Study the drawing (mm; zero at the part's minimum x, y, z) and answer. A direction names the side the tool comes from. Coordinates: 2 decimals unless noted, no trailing zeros. Order: outer loops, then holes, each group sorted by start corner. A loop starts at its lowest first (then second) coordinate and runs counter-clockwise, first axis right, second up.
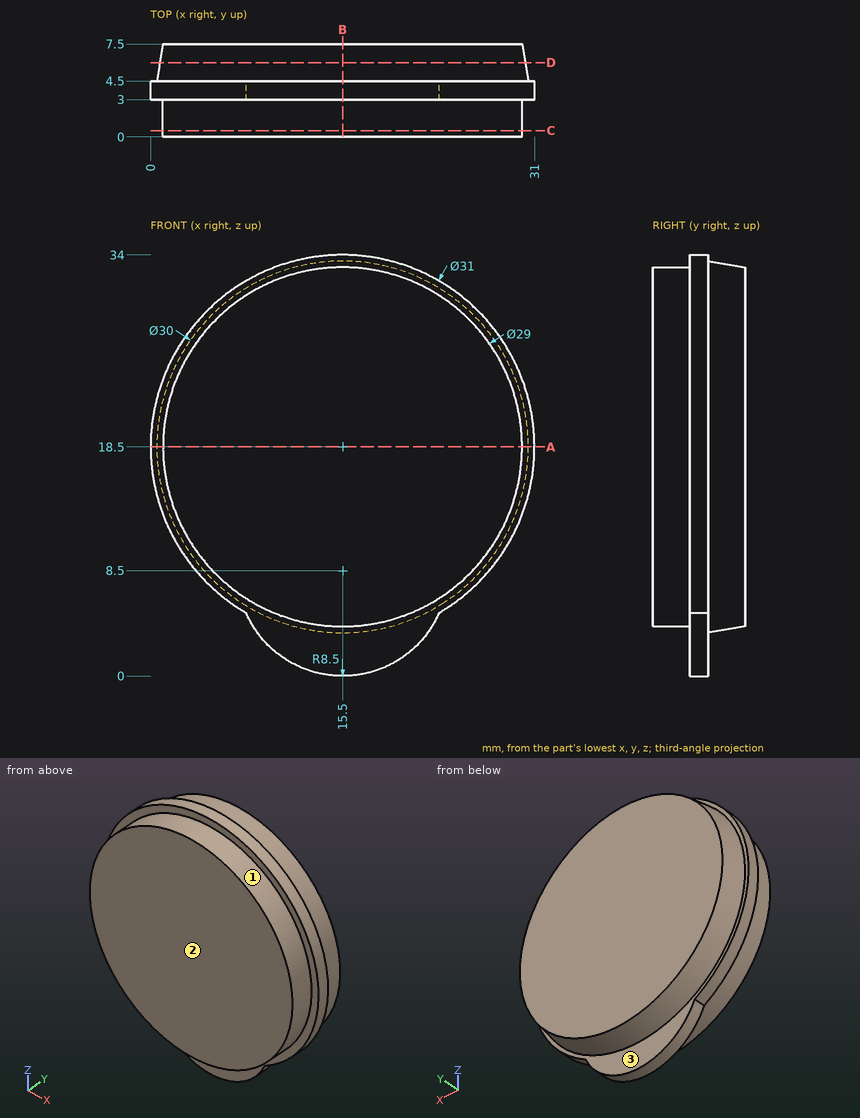
1) A cutting plane is placed at C-C, the plane y = 0.5. Determine the outline of the cut face in (x, z), and give its area (3 significant figures).
A:
outline: circle Ø29 at (15.5, 18.5)
area: 661 mm2
2) Straight lines are drawn through the part: line 1 (Y direction, x = 20, z = 2); line 2 (Z direction, x = 16, y = 0.75); line 3 (X direction, y = 7.25, z = 18). For each, find the intervals that lie inside material, in ascending order.
A:
line 1: y = 3 to 4.5
line 2: z = 4.01 to 32.99
line 3: x = 0.97 to 30.03
3) A cutting plane is placed at D-D, the plane y = 6. Determine the outline of the cut face in (x, z), and give its area (3 significant figures).
A:
outline: circle Ø29.5 at (15.5, 18.5)
area: 683 mm2
4) A cutting plane is placed at A-A, the plane z = 18.5. Determine the outline of the cut face in (x, y).
A:
outline: (0, 3) - (1, 3) - (1, 0) - (30, 0) - (30, 3) - (31, 3) - (31, 4.5) - (30.5, 4.5) - (30, 7.5) - (1, 7.5) - (0.5, 4.5) - (0, 4.5) - close
5) Flat-ended cylindrical pins translate along their axes: pin 1 Ø4 at (y, z) = (3.5, 14) entering from -X; pin 2 Ø3 at (x, y) = (9, 2.5) entering from +Z. Find the tip coordinate at first contact, or state that the pin passes through.
A:
pin 1: stops at x = 0.2
pin 2: stops at z = 33.14
6) A cutting plane is placed at B-B, the plane x = 15.5. Determine the outline of the cut face in (y, z).
A:
outline: (0, 4) - (3, 4) - (3, 0) - (4.5, 0) - (4.5, 3.5) - (7.5, 4) - (7.5, 33) - (4.5, 33.5) - (4.5, 34) - (3, 34) - (3, 33) - (0, 33) - close
7) Which of the six approach directions +Z, -Z, +X, -X, +Y, -Y give full straight-line access (tool end or side, diameter ignored) to the marked faces 1, 2 and 3?
A:
face 1: -Y
face 2: +Z, -Z, +X, -X, -Y
face 3: +Y
